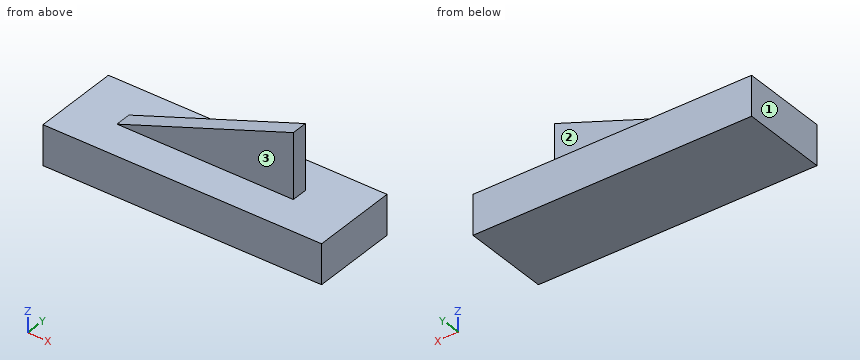
from build123d import *

# Parameters (mm, degrees)
F0_W          = 177.8
F0_H          = 55.496745
F1_DEPTH      = 25.4
F3_DEPTH      = 7.62
F3_DEPTH_BACK = 2.54


with BuildPart() as f1:
    # F0 (on Top) → F1 (new body)
    with BuildSketch(Plane.XY):
        with Locations((0.590887, -2.954431)):
            Rectangle(F0_W, F0_H)
    extrude(amount=F1_DEPTH)

    # F2 (on Front) → F3 (join, two sides)
    with BuildSketch(Plane.XZ) as f3_sk:
        Polygon((54.116055, 66.88869), (-58.625646, 25.348367), (54.116055, 25.078142), align=None)
    extrude(amount=F3_DEPTH)
    extrude(f3_sk.sketch, amount=-F3_DEPTH_BACK)


solid = f1.part
Could you check a few things on this model? Use its own coordinates, in mm. Face numbers are marked on the shaded views. A direction names the side the tool comes from. Give positions to 0.01 mm unless a question says otherwise; leave off trailing zeros. Write each loop counter-clockwise with the first axis right and the second up, starting at its lowest first coordinate (ties: lowest second). Pieces come first, ordered by that corner, then holes. Notation, with made-up numbers: (48, 40.25) -> (57, 40.25) arc R19 cw to (57, 62.25) -> close; hole circle Ø10 at (46, 20.5). An arc over 180 degrees is marked (long way). Answer as a JSON object with one key per item and string values.
Q1. Suppose I cut it at A-A on x = 22. Write out the boundary of the cut face in (y, z).
Taken from the geometry:
{"outline": "(-30.7, 0) -> (24.79, 0) -> (24.79, 25.4) -> (2.54, 25.4) -> (2.54, 55.06) -> (-7.62, 55.06) -> (-7.62, 25.4) -> (-30.7, 25.4) -> close"}
Q2. Suppose I cut it at B-B on y = 17. Write out the boundary of the cut face in (x, z).
Taken from the geometry:
{"outline": "(-88.31, 0) -> (89.49, 0) -> (89.49, 25.4) -> (-88.31, 25.4) -> close"}
Q3. Please list where these lines run through material, in increasing order: L1, parallel to Y at x = -34, z = 30.5; L2, parallel to Z at x = -67.5, y = -25.5; L3, parallel to Z at x = -51, y = 1.
Taken from the geometry:
{"L1": "y = -7.62 to 2.54", "L2": "z = 0 to 25.4", "L3": "z = 0 to 28.16"}
Q4. Suppose I cut it at D-D on z = 36.5. Write out the boundary of the cut face in (x, y), then the cut area to 3 significant figures.
Taken from the geometry:
{"outline": "(-28.36, -7.62) -> (54.12, -7.62) -> (54.12, 2.54) -> (-28.36, 2.54) -> close", "area": "838 mm²"}
Q5. Suppose I cut it at C-C on x = -53.5. Write out the boundary of the cut face in (y, z), then the cut area to 3 significant figures.
Taken from the geometry:
{"outline": "(-30.7, 0) -> (24.79, 0) -> (24.79, 25.4) -> (2.54, 25.4) -> (2.54, 27.24) -> (-7.62, 27.24) -> (-7.62, 25.4) -> (-30.7, 25.4) -> close", "area": "1,430 mm²"}
Q6. Which directions (+Z, -Z, +X, -X, +Y, -Y) give clear straight access to the entire face, cutting with the end or side of a thin tool? Please do the marked faces 1, 2 and 3.
Taken from the geometry:
{"face 1": "+Z, -Z, -X, +Y, -Y", "face 2": "+Z, +X, -X, +Y", "face 3": "+Z, +X, -X, -Y"}
Q7. Will these pins go through, and if not, where does the flat tip stop? pin 1 Ø10 at (x, y) = (55, 12.5) entering from +Z; pin 2 Ø20.5 at (x, z) = (-12, 45) entering from +Y; pin 3 Ø1.5 at (x, y) = (-46, -2) entering from +Z.
Taken from the geometry:
{"pin 1": "stops at z = 25.4", "pin 2": "stops at y = 2.54", "pin 3": "stops at z = 30.28"}
